Geometry check sheet. Reference: the model listing, model coordinates, mm. Give positions to 0.01 mm unless a question says otherwise; leave off trailing zeros. Write each loop counter-clockwise with the first axis right and the second up, starting at its lowest first coordinate (ties: lowest second). Pieces come first, ordered by that corner, then holes. Notation, with made-up numbers: (39.25, -1.75) - (77.25, -1.75) arc R23 ccw to (77.25, 19.25) - close; hole circle Ø4 at (64, 52). An arc over 180 degrees is marked (long way). Write item = value, one per line. Start each with the question number.
(1) Section check A-A, the plane z = 1.75. Give the number of separate pieces and of enclosed holes in the cut face, plus the area to 3 significant figures.
(2) Section check C-C, the plane x = 38.5. Enter the section's corners in (y, z), plus the area to 3 significant figures.
(3) Thickness scan on L1, parallel to X at y = 33, z = 2.2; L2, parallel to Y at x = 23.5, z = 0.6; L3, parallel to Y at x = 15, z = 1. Record the ranges inside material, lowest first.
(4) Section check B-B, the plane y = -78.5. Enter the section's corners in (x, z).
(5) Depth check by flat-ended pin: pin 1 Ø0.8 at (x, z) = (-30.5, 2) entering from +Y; pin 2 Ø1 at (x, z) = (42.5, 1.5) entering from -Y; pin 3 Ø1.2 at (y, z) = (41, 1) entering from +X. Enter the tip coordinate at first touch or a pass-through.
(6) Draft check along Y on faces 1 (the cylindrical face through (-15, -82, 1)), 2 (the cylindrical face through (-0.8, -101.24, 1.23)), 3 (the flat face through (1, 9, 0)). Enter one of: pulls with the +Y half, pulls with the -Y half, needs draft (parallel to the pull), parting line crosses it, or undercut.
```python
from build123d import *

# Parameters (mm, degrees)
PAD_DEPTH       = 2.5
SKETCH001_W     = 3
SKETCH001_H     = 11.5
POCKET_DEPTH    = 2.501
FILLET_R        = 2
FILLET001_R     = 2
SKETCH002_W     = 6
SKETCH002_H     = 20
POCKET001_DEPTH = 2.501
SKETCH003_R     = 2
POCKET002_DEPTH = 2.501
POCKET003_DEPTH = 2.501


with BuildPart() as part:
    # Sketch → Pad (new body)
    with BuildSketch(Plane.XY):
        with BuildLine():
            Line((55, 85), (55, -85))
            ThreePointArc((-55, -85), (0, -101.242284), (55, -85))
            Line((-55, -85), (-55, 85))
            Line((-55, 85), (-80, 85))
            ThreePointArc((80, 85), (0, 116.726175), (-80, 85))
            Line((80, 85), (55, 85))
        make_face()
    extrude(amount=PAD_DEPTH)

    # Sketch001 → Pocket (cut, through all)
    with BuildSketch(Plane.XY.offset(2.5)):
        with Locations((-53.5, 15.75)):
            Rectangle(SKETCH001_W, SKETCH001_H)
        with Locations((53.5, 15.75)):
            Rectangle(SKETCH001_W, SKETCH001_H)
        with Locations((-30.5, 15.75)):
            Rectangle(SKETCH001_W, SKETCH001_H)
        with Locations((30.5, 15.75)):
            Rectangle(SKETCH001_W, SKETCH001_H)
    extrude(amount=-POCKET_DEPTH, mode=Mode.SUBTRACT)

    # Fillet
    fillet_edges = [part.edges().sort_by_distance(p)[0] for p in [
        (-55, 85, 1.25),
        (55, 85, 1.25),
    ]]
    fillet(fillet_edges, radius=FILLET_R)

    # Fillet001
    fillet001_edges = [part.edges().sort_by_distance(p)[0] for p in [
        (80, 85, 1.25),
        (-80, 85, 1.25),
        (-55, -85, 1.25),
        (55, -85, 1.25),
    ]]
    fillet(fillet001_edges, radius=FILLET001_R)

    # Sketch002 → Pocket001 (cut, through all)
    with BuildSketch(Plane.XY.offset(2.5)):
        with Locations((-25, 36.5)):
            Rectangle(SKETCH002_W, SKETCH002_H)
        with Locations((25, 36.5)):
            Rectangle(SKETCH002_W, SKETCH002_H)
    extrude(amount=-POCKET001_DEPTH, mode=Mode.SUBTRACT)

    # Sketch003 → Pocket002 (cut, through all)
    with BuildSketch(Plane.XY.offset(2.5)):
        with Locations((-15, -60)):
            Circle(SKETCH003_R)
        with Locations((15, -60)):
            Circle(SKETCH003_R)
        with Locations((15, -84)):
            Circle(SKETCH003_R)
        with Locations((-15, -84)):
            Circle(SKETCH003_R)
    extrude(amount=-POCKET002_DEPTH, mode=Mode.SUBTRACT)

    # Sketch004 → Pocket003 (cut, through all)
    with BuildSketch(Plane.XY.offset(2.5)):
        with BuildLine():
            ThreePointArc((-25, -23), (-27, -25), (-25, -27))
            Line((-25, -27), (-14, -27))
            ThreePointArc((-14, -27), (-12, -25), (-14, -23))
            Line((-25, -23), (-14, -23))
        make_face()
        with BuildLine():
            ThreePointArc((14, -23), (12, -25), (14, -27))
            Line((14, -27), (25, -27))
            ThreePointArc((25, -27), (27, -25), (25, -23))
            Line((14, -23), (25, -23))
        make_face()
    extrude(amount=-POCKET003_DEPTH, mode=Mode.SUBTRACT)


solid = part.part
```
Model answer:
q1.separate_pieces = 1
q1.enclosed_holes = 10
q1.area = 22,800 mm²
q2.outline = (-93.64, 0) - (110.19, 0) - (110.19, 2.5) - (-93.64, 2.5) - close
q2.area = 510 mm²
q3.L1 = -55 to -28, -22 to 22, 28 to 55
q3.L2 = -98.48 to -27, -23 to 26.5, 46.5 to 114.34
q3.L3 = -100.12 to -86, -82 to -62, -58 to -27, -23 to 115.76
q4.outline = (-55, 0) - (55, 0) - (55, 2.5) - (-55, 2.5) - close
q5.pin_1 = 112.78
q5.pin_2 = -92.12
q5.pin_3 = 55
q6.face_1 = undercut
q6.face_2 = pulls with the -Y half
q6.face_3 = needs draft
